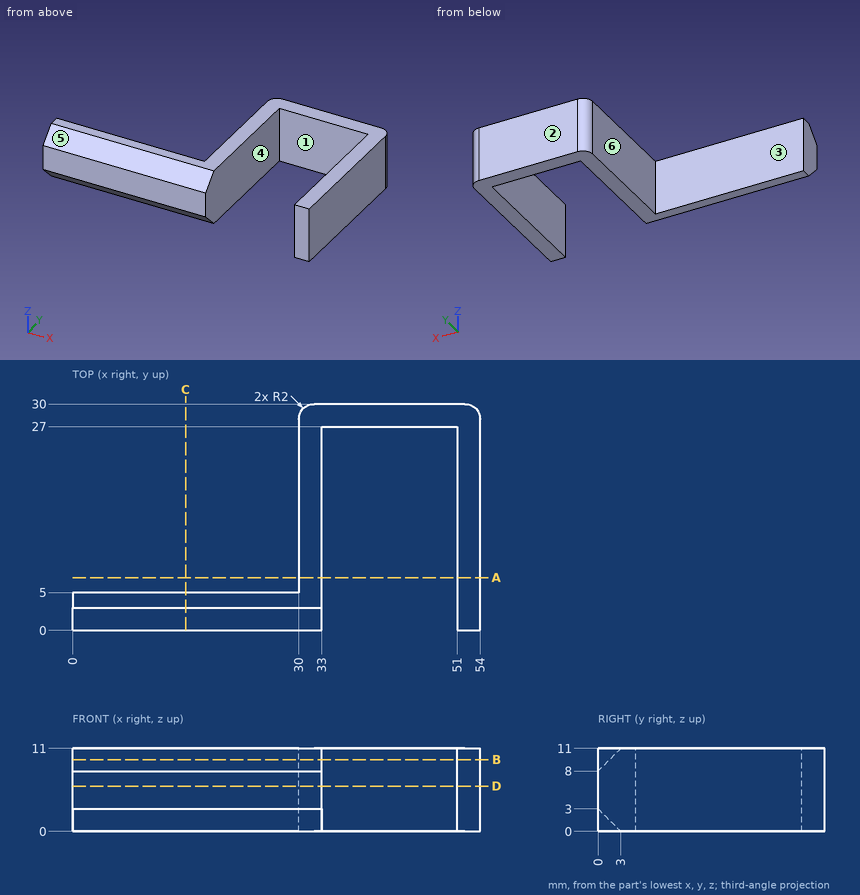
Answer from the drawing. Dimensions are ordinates in mm from the lowest x, y and z of the part. A direction names the side the tool comes from. Coordinates: 2 decimals unless noted, no trailing zeros. Write each loop counter-clockwise with the first axis right and the second up, starting at its lowest first coordinate (ties: lowest second). Pieces come first, ordered by that corner, then holes. Notation, with made-up numbers: (58.5, -38) - (104.5, -38) arc R10 cw to (104.5, -22) - close; hole circle Ø4 at (-14.5, 82). An arc over 180 degrees is marked (long way). One line per question, with ' | ' between items.
Q1. Find section B-B, the plane z = 9.5. Write down the section's boundary in (x, y).
Result set:
outline: (0, 1.5) - (33, 1.5) - (33, 27) - (51, 27) - (51, 0) - (54, 0) - (54, 28) arc R2 ccw to (52, 30) - (32, 30) arc R2 ccw to (30, 28) - (30, 5) - (0, 5) - close
Q2. Find section C-C, the plane x = 15. Write down the section's boundary in (y, z), plus the area to 3 significant figures.
Result set:
outline: (0, 3) - (3, 0) - (5, 0) - (5, 11) - (3, 11) - (0, 8) - close | area: 46.0 mm^2
Q3. Determine the mould class of the marked faces 4, 5 and 6 for opening direction X: +X half, -X half, draft (parallel to the pull), parting line (faces both ways), or undercut.
Result set:
face 4: undercut | face 5: draft | face 6: -X half
Q4. Find section D-D, the plane z = 6. Write down the section's boundary in (x, y), plus the area to 3 significant figures.
Result set:
outline: (0, 0) - (33, 0) - (33, 27) - (51, 27) - (51, 0) - (54, 0) - (54, 28) arc R2 ccw to (52, 30) - (32, 30) arc R2 ccw to (30, 28) - (30, 5) - (0, 5) - close | area: 382 mm^2
Q5. For the marked faces 1, 2 and 3, determine the directions among +Z, -Z, +X, -X, +Y, -Y from which every point of the face is accessible in a straight line to the end or side of a thin tool.
Result set:
face 1: +Z, -Z, -Y | face 2: +Z, -Z, +X, -X, +Y | face 3: +Z, -Z, -X, +Y
Q6. Find section A-A, the plane y = 7. Write down the section's boundary in (x, z), plus the area to 3 significant figures.
Result set:
outline: (30, 0) - (33, 0) - (33, 11) - (30, 11) - close; (51, 0) - (54, 0) - (54, 11) - (51, 11) - close | area: 66.0 mm^2
Q7. Consider L1, parallel to X at y = 20.5, z = 9; L2, parallel to X at y = 2.5, z = 7.5; L3, parallel to Y at x = 41, z = 5. Determine where each line is inside the solid, lowest interval first. Write a range as [from, to].
Result set:
L1: [30, 33], [51, 54] | L2: [0, 33], [51, 54] | L3: [27, 30]
Q8. Each of these flat-tipped pins is pushed along its axis until it touches: P1, Ø5.5, axis at y = 11.5, z = 5.5, coming from the -X side; P2, Ø10, axis at x = 27.5, y = 20, coming from the -Z side; P3, Ø3.5, axis at x = 10.5, z = 6, coming from the +Y side. Where does it stop, or does it pass through?
Result set:
P1: x = 30 | P2: z = 0 | P3: y = 5
